```python
from build123d import *

# Parameters (mm, degrees)
F2_DEPTH = 5


with BuildPart() as f2:
    # F1 (on Right) → F2 (new body)
    with BuildSketch(Plane.YZ):
        Polygon((-71.5, 15), (0, 0), (0, 7.1), (4, 7.1), (4, 12.9), (0, 12.9), (0, 20), (-5, 20), (-5, 25), (-15, 25), (-15, 20), (-18.4, 20), (-18.4, 17.5), (-17.25, 17.5), (-17.25, 15), (-20, 15), (-22.75, 15), (-22.75, 17.5), (-21.6, 17.5), (-21.6, 20), (-25, 20), (-25, 25), (-45, 25), (-45, 20), (-48.4, 20), (-48.4, 17.5), (-47.25, 17.5), (-47.25, 15), (-50, 15), (-52.75, 15), (-52.75, 17.5), (-51.6, 17.5), (-51.6, 20), (-55, 20), (-55, 25), (-65, 25), (-65, 20), (-71.5, 20), align=None)
    extrude(amount=F2_DEPTH)


solid = f2.part
```
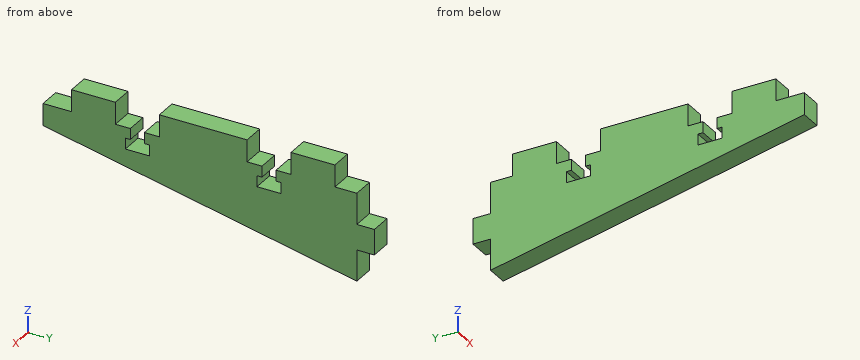
Here's how the part is built. I have some questions about the finished solid (model axes, mm). Round coordinates to 2 decimals unless told otherwise and drop trailing zeros. Loops run counter-clockwise (first coordinate to the right, second up) from the corner with the lowest first, then second, coordinate; pieces in that order, holes last. Notation, with made-up numbers: (-23, 68.25) -> (5, 68.25) arc R38 cw to (5, 107.25) -> close; hole circle Ø7 at (43, 76.25). An arc over 180 degrees is marked (long way). Answer as CSV lines item,"result". Start each with the question number.
1. Imagine slicing it at A-A on z = 18.5. Write out the boundary of the cut face in (x, y), plus the area to 4 significant figures.
2. I'm going to push flat-ended pins straight in: P1, Ø1.7, axis at x = 3, y = -46, coming from the +Z side; P2, Ø1.3, axis at x = 3.5, y = -18, coming from the -Z side; P3, Ø1.5, axis at x = 3.5, y = -49.5, coming from the +Z side. Where does each tip first touch, or does it pass through?
3. Imagine slicing it at B-B on z = 23. Write out the boundary of the cut face in (x, y).
4. I need wall thicknesses on probe 1 along Y at (x, z) = (2.95, 19); probe 2 along Y at (x, z) = (1.75, 21.5); probe 3 along Z at (x, y) = (3.2, -8). Which ranges of each line are inside material? Lowest first, please. Write a range as from..to.
5. Imagine slicing it at D-D on y = -39. Write out the boundary of the cut face in (x, z), plus the area to 3 significant figures.
6. Imagine slicing it at C-C on z = 3. Write out the boundary of the cut face in (x, y).
Solution:
1,outline,"(0, -71.5) -> (5, -71.5) -> (5, -51.6) -> (0, -51.6) -> close; (0, -48.4) -> (5, -48.4) -> (5, -21.6) -> (0, -21.6) -> close; (0, -18.4) -> (5, -18.4) -> (5, 0) -> (0, 0) -> close"
1,area,"325.5 mm²"
2,P1,"z = 20"
2,P2,"z = 3.64"
2,P3,"z = 15"
3,outline,"(0, -65) -> (5, -65) -> (5, -55) -> (0, -55) -> close; (0, -45) -> (5, -45) -> (5, -25) -> (0, -25) -> close; (0, -15) -> (5, -15) -> (5, -5) -> (0, -5) -> close"
4,probe 1,"-71.5..-51.6, -48.4..-21.6, -18.4..0"
4,probe 2,"-65..-55, -45..-25, -15..-5"
4,probe 3,"1.68..25"
5,outline,"(0, 8.18) -> (5, 8.18) -> (5, 25) -> (0, 25) -> close"
5,area,"84.1 mm²"
6,outline,"(0, -14.3) -> (5, -14.3) -> (5, 0) -> (0, 0) -> close"
